Part model, mm, in its own coordinate system. A direction names the side the tool comes from. Round coordinates to 2 decimals unless told otherwise and drop trailing zeros. Order: outer loops, then holes, each group sorted by start corner. A loop starts at its lowest first (then second) coordinate and runs counter-clockwise, first axis right, second up. Notation, with made-up numbers: M 20,-0.5 L 78,-0.5 A23 ccw 78,12.5 Z; hole C 88,76.5 d9. An arc over 180 degrees is marked long. One line per question, with ' | ' between items.
from build123d import *

# Parameters (mm, degrees)
F0_W     = 145
F0_H     = 75
F0_R     = 1.5
F0_R_2   = 4
F1_DEPTH = 3
F2_R     = 7
F3_DEPTH = 2


with BuildPart() as f1:
    # F0 (on Top) → F1 (new body)
    with BuildSketch(Plane.XY):
        with Locations((72.5, -37.5)):
            Rectangle(F0_W, F0_H)
        with Locations((5.110198, -63.145563)):
            Circle(F0_R, mode=Mode.SUBTRACT)
        with Locations((45.909047, -45.651395)):
            Circle(F0_R_2, mode=Mode.SUBTRACT)
        with Locations((141.360894, -63.145511)):
            Circle(F0_R, mode=Mode.SUBTRACT)
        with Locations((107.167281, -45.651395)):
            Circle(F0_R_2, mode=Mode.SUBTRACT)
        with Locations((45.909047, -24.54808)):
            Circle(F0_R_2, mode=Mode.SUBTRACT)
        with Locations((5.110172, -12.241635)):
            Circle(F0_R, mode=Mode.SUBTRACT)
        with Locations((107.167281, -24.54808)):
            Circle(F0_R_2, mode=Mode.SUBTRACT)
        with Locations((141.062453, -12.241724)):
            Circle(F0_R, mode=Mode.SUBTRACT)
    extrude(amount=F1_DEPTH)

    # F2 (on face) → F3 (cut)
    with BuildSketch(Plane.XY.offset(3)):
        with BuildLine():
            Line((-4.892084, -14.741702), (5.110175, -14.741702))
            ThreePointArc((5.110175, -14.741702), (7.610175, -12.241702), (5.110175, -9.741702))
            Line((5.110175, -9.741702), (-4.892084, -9.741702))
            Line((-4.892084, -9.741702), (-4.892084, -14.741702))
        make_face()
        with BuildLine():
            Line((-4.892084, -65.645501), (5.110175, -65.645501))
            ThreePointArc((5.110175, -65.645501), (7.610175, -63.145501), (5.110175, -60.645501))
            Line((5.110175, -60.645501), (-4.892084, -60.645501))
            Line((-4.892084, -60.645501), (-4.892084, -65.645501))
        make_face()
        with BuildLine():
            Line((149.460912, -9.741702), (141.062498, -9.741702))
            ThreePointArc((141.062498, -9.741702), (138.562498, -12.241702), (141.062498, -14.741702))
            Line((141.062498, -14.741702), (149.460912, -14.741702))
            Line((149.460912, -14.741702), (149.460912, -9.741702))
        make_face()
        with BuildLine():
            Line((150.567517, -60.645501), (141.360864, -60.645501))
            ThreePointArc((141.360864, -60.645501), (138.860864, -63.145501), (141.360864, -65.645501))
            Line((141.360864, -65.645501), (150.567517, -65.645501))
            Line((150.567517, -65.645501), (150.567517, -60.645501))
        make_face()
        with Locations((45.909047, -24.54808)):
            Circle(F2_R)
        with Locations((45.909047, -45.651395)):
            Circle(F2_R)
        with Locations((107.167281, -24.54808)):
            Circle(F2_R)
        with Locations((107.167281, -45.651395)):
            Circle(F2_R)
    extrude(amount=-F3_DEPTH, mode=Mode.SUBTRACT)


solid = f1.part
1) Two-plate mould, pull along Y, no slides. Class faces 5 (the face through (49.724, -23.347, 0.493)), 6 (the face through (103.17, -24.37, 0.49)), 7 (the face through (71, -37, 3)), 8 (the face through (71, 0, 1)): released by +Y, released by -Y, zero draft, split by the parting line, or undercut.
The answers:
face 5: undercut | face 6: undercut | face 7: zero draft | face 8: released by +Y
2) Probe line 1 (X direction, y = -45, z = 2.8); line 2 (Y direction, x = 107, z = 0.6); line 3 (X direction, y = -48.5, z = 0.5). List the from-to ranges inside material, lowest first. Write a range as [from, to].
The answers:
line 1: x = [0, 38.94], [52.88, 100.2], [114.14, 145] | line 2: y = [-75, -49.65], [-41.65, -28.54], [-20.55, 0] | line 3: x = [0, 43.1], [48.72, 104.36], [109.98, 145]
3) Which spindle directions (+Z, -Z, +X, -X, +Y, -Y) get a long thin tool onto all of the face, cutting with end or side? Do faces 1 (the face through (7.61, -12.3, 2.01)), 2 (the face through (106.647, -41.685, 0.493)), 3 (the face through (52.375, -48.332, 2.014)), 4 (the face through (143.3, -63.1, 1)). Say none if no direction does.
The answers:
face 1: +Z, -X | face 2: +Z, -Z | face 3: +Z | face 4: +Z, +X
4) Saw through at A-A (y = -26.5). List the corners of the cut face in (x, z).
The answers:
outline: M 0,0 L 42.42,0 L 42.42,1 L 39.19,1 L 39.19,3 L 0,3 Z; M 49.4,0 L 103.68,0 L 103.68,1 L 100.44,1 L 100.44,3 L 52.63,3 L 52.63,1 L 49.4,1 Z; M 110.66,0 L 145,0 L 145,3 L 113.89,3 L 113.89,1 L 110.66,1 Z
5) Saw through at C-C (z = 2.15). List the corners of the cut face in (x, y).
The answers:
outline: M 0,-75 L 145,-75 L 145,-65.65 L 141.36,-65.65 A2.5 cw 141.36,-60.65 L 145,-60.65 L 145,-14.74 L 141.06,-14.74 A2.5 cw 141.06,-9.74 L 145,-9.74 L 145,0 L 0,0 L 0,-9.74 L 5.11,-9.74 A2.5 cw 5.11,-14.74 L 0,-14.74 L 0,-60.65 L 5.11,-60.65 A2.5 cw 5.11,-65.65 L 0,-65.65 Z; hole C 45.91,-45.65 d14; hole C 45.91,-24.55 d14; hole C 107.17,-45.65 d14; hole C 107.17,-24.55 d14
6) Drop a flat-ended pin along its axis: pin 1 (4 mm diameter, centred on x = 48.5, y = -28, fed in from +Z). Give the stop position or say it passes through.
The answers:
pin 1: stops at z = 1
7) Saw through at B-B (x = 45.5). List the corners of the cut face in (y, z), plus the area to 3 significant figures.
The answers:
outline: M -75,0 L -49.63,0 L -49.63,1 L -52.64,1 L -52.64,3 L -75,3 Z; M -41.67,0 L -28.53,0 L -28.53,1 L -31.54,1 L -31.54,3 L -38.66,3 L -38.66,1 L -41.67,1 Z; M -20.57,0 L 0,0 L 0,3 L -17.56,3 L -17.56,1 L -20.57,1 Z | area: 153 mm²
